```python
from build123d import *

# Parameters (mm, degrees)
SKETCH_1_W          = 45
SKETCH_1_H          = 45
SKETCH_1_R          = 1.6
EXTRUDE_1_DEPTH     = 3
SKETCH_2_W          = 8.01
SKETCH_2_H          = 3.01
CUT_EXTRUDE_1_DEPTH = 3
SKETCH_4_R          = 1
SKETCH_4_R_2        = 1.6
CUT_EXTRUDE_2_DEPTH = 3
SKETCH_5_W          = 28
SKETCH_5_H          = 18
CUT_EXTRUDE_3_DEPTH = 3
CHAMFER_1_SIZE      = 4
FILLET_1_R          = 2


with BuildPart() as part:
    # 草图1 → 凸台-拉伸1 (new body)
    with BuildSketch(Plane(origin=(0, 0, 0), x_dir=(1, 0, 0), z_dir=(0, 1, 0))):
        Rectangle(SKETCH_1_W, SKETCH_1_H)
        with Locations(Location((19, 0, 0), (0, 0, 270))):
            Circle(SKETCH_1_R, mode=Mode.SUBTRACT)
        with Locations(Location((-19, 0, 0), (0, 0, 270))):
            Circle(SKETCH_1_R, mode=Mode.SUBTRACT)
    extrude(amount=EXTRUDE_1_DEPTH)

    # 草图2 → 切除-拉伸1 (cut)
    with BuildSketch(Plane(origin=(0, 3, 0), x_dir=(1, 0, 0), z_dir=(0, 1, 0))):
        with Locations((-11.005, -17.5)):
            Rectangle(SKETCH_2_W, SKETCH_2_H)
        with Locations((11.005, -17.5)):
            Rectangle(SKETCH_2_W, SKETCH_2_H)
        with Locations((-11.005, 17.5)):
            Rectangle(SKETCH_2_W, SKETCH_2_H)
        with Locations((11.005, 17.5)):
            Rectangle(SKETCH_2_W, SKETCH_2_H)
    extrude(amount=-CUT_EXTRUDE_1_DEPTH, mode=Mode.SUBTRACT)

    # 草图4 → 切除-拉伸2 (cut)
    with BuildSketch(Plane(origin=(0, 3, 0), x_dir=(1, 0, 0), z_dir=(0, 1, 0))):
        with Locations((-14.01, -15.995)):
            Circle(SKETCH_4_R)
        with Locations((-14.01, -19.005)):
            Circle(SKETCH_4_R)
        with Locations((-8, -15.995)):
            Circle(SKETCH_4_R)
        with Locations((-8, -19.005)):
            Circle(SKETCH_4_R)
        with Locations((8, -19.005)):
            Circle(SKETCH_4_R)
        with Locations((8, -15.995)):
            Circle(SKETCH_4_R)
        with Locations((14.01, -19.005)):
            Circle(SKETCH_4_R)
        with Locations((14.01, -15.995)):
            Circle(SKETCH_4_R)
        with Locations((-8, 19.005)):
            Circle(SKETCH_4_R)
        with Locations((-8, 15.995)):
            Circle(SKETCH_4_R)
        with Locations((-14.01, 19.005)):
            Circle(SKETCH_4_R)
        with Locations((-14.01, 15.995)):
            Circle(SKETCH_4_R)
        with Locations((14.01, 15.995)):
            Circle(SKETCH_4_R)
        with Locations((14.01, 19.005)):
            Circle(SKETCH_4_R)
        with Locations((8, 15.995)):
            Circle(SKETCH_4_R)
        with Locations((8, 19.005)):
            Circle(SKETCH_4_R)
        with Locations(Location((0, -13, 0), (0, 0, 270))):
            Circle(SKETCH_4_R_2)
        with Locations(Location((0, 13, 0), (0, 0, 90))):
            Circle(SKETCH_4_R_2)
    extrude(amount=-CUT_EXTRUDE_2_DEPTH, mode=Mode.SUBTRACT)

    # 草图5 → 切除-拉伸3 (cut)
    with BuildSketch(Plane(origin=(0, 3, 0), x_dir=(1, 0, 0), z_dir=(0, 1, 0))):
        Rectangle(SKETCH_5_W, SKETCH_5_H)
    extrude(amount=-CUT_EXTRUDE_3_DEPTH, mode=Mode.SUBTRACT)

    # 倒角1
    chamfer_1_edges = [part.edges().sort_by_distance(p)[0] for p in [
        (14, 1.5, -9),
        (14, 1.5, 9),
        (-14, 1.5, 9),
        (-14, 1.5, -9),
        (22.5, 1.5, 22.5),
        (-22.5, 1.5, 22.5),
        (-22.5, 1.5, -22.5),
        (22.5, 1.5, -22.5),
    ]]
    chamfer(chamfer_1_edges, length=CHAMFER_1_SIZE)

    # 圆角1
    fillet_1_edges = [part.edges().sort_by_distance(p)[0] for p in [
        (-22.5, 1.5, 18.5),
        (-22.5, 1.5, -18.5),
        (18.5, 1.5, -22.5),
        (-18.5, 1.5, -22.5),
        (22.5, 1.5, 18.5),
        (22.5, 1.5, -18.5),
        (-18.5, 1.5, 22.5),
        (18.5, 1.5, 22.5),
        (10, 1.5, 9),
        (-10, 1.5, 9),
        (-14, 1.5, -5),
        (-14, 1.5, 5),
        (14, 1.5, -5),
        (14, 1.5, 5),
        (-10, 1.5, -9),
        (10, 1.5, -9),
    ]]
    fillet(fillet_1_edges, radius=FILLET_1_R)


solid = part.part
```
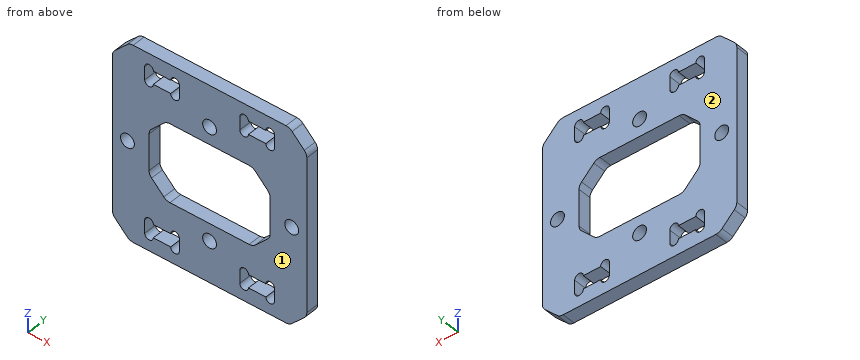
Can you work these out from the model? Positions are in its coordinate system, mm. Face numbers are marked on the shaded views. Coordinates: 2 decimals unless noted, no trailing zeros. Write each loop counter-clockwise with the first axis right and the second up, starting at its lowest first coordinate (ties: lowest second). Pieces come first, ordered by that corner, then holes. Notation, with made-up numbers: M 49.5,-23 L 90.5,-23 A27 ccw 90.5,-1 Z; hole C 33,88 d4. An arc over 180 degrees is marked long. Write item = value, one per line. Start each with the question number.
Q1. If we section it at B-B, the plane x = 0: Write out the boundary of the cut face in (y, z).
Q2. If I drill on L1, parallel to X at y = 2.35, z = 17.5; L2, parallel to X at y = 1.05, z = 0; L3, parallel to X at y = 1.6, z = 13, over which ranges is the centre line in solid material (lowest first)? Write a range as [from, to].
Q3. If we section it at D-D, the plane y = 2: State how many separate pieces and enclosed holes the cut face has, then the cut area to 3 significant figures.
Q4. If we section it at A-A, the plane z = 0: Write out the boundary of the cut face in (x, y).
Q5. Thinking about a two-plate mould opening in Y: for the marked faces 1 and 2, which applies, released by +Y, released by -Y, zero draft, split by the parting line, or undercut?
Q6. If we section it at C-C, the plane z = 13: Write out the boundary of the cut face in (x, y), then the cut area to 3 significant figures.
Check sheet entries:
q1.outline = M 0,-22.5 L 3,-22.5 L 3,-14.6 L 0,-14.6 Z; M 0,-11.4 L 3,-11.4 L 3,-9 L 0,-9 Z; M 0,9 L 3,9 L 3,11.4 L 0,11.4 Z; M 0,14.6 L 3,14.6 L 3,22.5 L 0,22.5 Z
q2.L1 = [-22.5, -15.01], [-7, 7], [15.01, 22.5]
q2.L2 = [-22.5, -20.6], [-17.4, -14], [14, 17.4], [20.6, 22.5]
q2.L3 = [-22.5, -1.6], [1.6, 22.5]
q3.separate_pieces = 1
q3.enclosed_holes = 9
q3.area = 1,370 mm²
q4.outline = M -22.5,0 L -20.6,0 L -20.6,3 L -22.5,3 Z; M -17.4,0 L -14,0 L -14,3 L -17.4,3 Z; M 14,0 L 17.4,0 L 17.4,3 L 14,3 Z; M 20.6,0 L 22.5,0 L 22.5,3 L 20.6,3 Z
q5.face_1 = released by -Y
q5.face_2 = released by +Y
q6.outline = M -22.5,0 L -1.6,0 L -1.6,3 L -22.5,3 Z; M 1.6,0 L 22.5,0 L 22.5,3 L 1.6,3 Z
q6.area = 125 mm²
